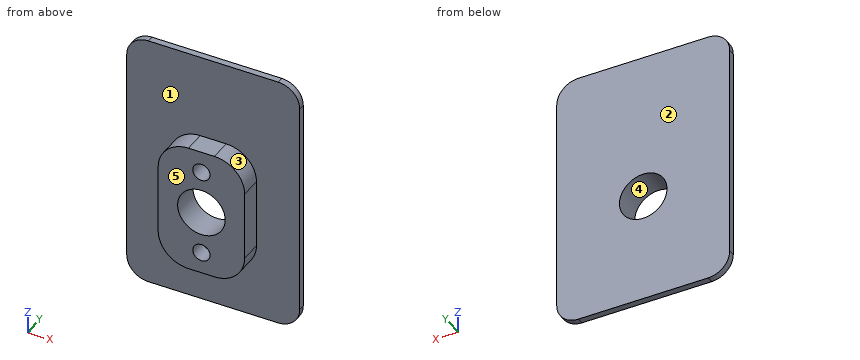
```python
from build123d import *

# Parameters (mm, degrees)
F0_W     = 40
F0_H     = 60
F0_R     = 5.5
F1_DEPTH = 1.5
F2_W     = 20
F2_H     = 30
F2_R     = 5.5
F3_DEPTH = 5
F4_R     = 2
F5_DEPTH = 4
F6_R     = 7
F7_R     = 5


with BuildPart() as f1:
    # F0 (on Front) → F1 (new body)
    with BuildSketch(Plane.XZ):
        with Locations((0, 4.5)):
            Rectangle(F0_W, F0_H)
        Circle(F0_R, mode=Mode.SUBTRACT)
    extrude(amount=F1_DEPTH)

    # F2 (on face) → F3 (join)
    with BuildSketch(Plane.XZ.offset(1.5)):
        Rectangle(F2_W, F2_H)
        Circle(F2_R, mode=Mode.SUBTRACT)
    extrude(amount=F3_DEPTH)

    # F4 (on face) → F5 (cut)
    with BuildSketch(Plane.XZ.offset(6.5)):
        with Locations((0, 10)):
            Circle(F4_R)
        with Locations((0, -10)):
            Circle(F4_R)
    extrude(amount=-F5_DEPTH, mode=Mode.SUBTRACT)

    # F6
    f6_edges = [f1.edges().sort_by_distance(p)[0] for p in [
        (10, -4, 15),
        (-10, -4, 15),
        (10, -4, -15),
        (-10, -4, -15),
    ]]
    fillet(f6_edges, radius=F6_R)

    # F7
    f7_edges = [f1.edges().sort_by_distance(p)[0] for p in [
        (20, -0.75, 34.5),
        (20, -0.75, -25.5),
        (-20, -0.75, -25.5),
        (-20, -0.75, 34.5),
    ]]
    fillet(f7_edges, radius=F7_R)


solid = f1.part
```
Input: part model. Units: mm. Frame: model coordinates. Face numbers are marked on the shaded views. A direction names the side the tool comes from. Round coordinates to 2 decimals unless told otherwise and drop trailing zeros. Loops run counter-clockwise (first coordinate to the right, second up) from the corner with the lowest first, then second, coordinate; pieces in that order, holes last. Notation, with made-up numbers: (39, 72) - (96, 72) arc R29 cw to (96, 99) - close; hole circle Ø6 at (74.25, -32.75). An arc over 180 degrees is marked (long way). One line per item, written item: value. Start each with the question number.
(1) Section B-B, the plane y = -3.25. Return loops of the section in (x, z).
(2) Access query for the marked faces 1 and 2. Directions: +Z, -Z, +X, -X, +Y, -Y. A direction counts if a zero-diameter tool reaches every point of the face in a straight line with its end or side. Return the directions, or none.
(3) Ray query, line 1 (Z direction, x = 0, y = -3.6); line 2 (Y direction, x = -5, z = 19); line 3 (X direction, y = -4.75, z = 1). Return the intervals inside material, ascending. Write a range as [from, to].
(4) Section D-D, the plane x = -8. Return loops of the section in (y, z).
(5) Draft query along Z for the marked faces 3, 4 and 5. Return one class per face: +Z half, -Z half, draft (parallel to the pull), parting line (faces both ways), or undercut.
(6) Contact query for flat-ended pins moving along their axis: P1, Ø9, axis at x = 0, z = 0, coming from the +Y side; P2, Ø1.5, axis at y = -3.5, z = -2.5, coming from the -X side; P3, Ø2, axis at x = 6.5, y = -3, coming from the -Z side. Output: stop coordinate, or through.
(7) Section A-A, the plane z = 0. Return loops of the section in (x, y).
(8) Section C-C, the plane x = 0. Return loops of the section in (y, z), plus the area to 4 significant figures.
Results below:
1. outline: (-10, -8) arc R7 ccw to (-3, -15) - (3, -15) arc R7 ccw to (10, -8) - (10, 8) arc R7 ccw to (3, 15) - (-3, 15) arc R7 ccw to (-10, 8) - close; hole circle Ø11 at (0, 0); hole circle Ø4 at (0, -10); hole circle Ø4 at (0, 10)
2. face 1: -Y
2. face 2: +Z, -Z, +X, -X, +Y
3. line 1: [-15, -12], [-8, -5.5], [5.5, 8], [12, 15]
3. line 2: [-1.5, 0]
3. line 3: [-10, -5.41], [5.41, 10]
4. outline: (-6.5, -12.9) - (-1.5, -12.9) - (-1.5, -25.5) - (0, -25.5) - (0, 34.5) - (-1.5, 34.5) - (-1.5, 12.9) - (-6.5, 12.9) - close
5. face 3: +Z half
5. face 4: undercut
5. face 5: draft
6. P1: through
6. P2: x = -10
6. P3: z = -14.54
7. outline: (-20, -1.5) - (-10, -1.5) - (-10, -6.5) - (-5.5, -6.5) - (-5.5, 0) - (-20, 0) - close; (5.5, -6.5) - (10, -6.5) - (10, -1.5) - (20, -1.5) - (20, 0) - (5.5, 0) - close
8. outline: (-6.5, -15) - (-1.5, -15) - (-1.5, -25.5) - (0, -25.5) - (0, -5.5) - (-6.5, -5.5) - (-6.5, -8) - (-2.5, -8) - (-2.5, -12) - (-6.5, -12) - close; (-6.5, 5.5) - (0, 5.5) - (0, 34.5) - (-1.5, 34.5) - (-1.5, 15) - (-6.5, 15) - (-6.5, 12) - (-2.5, 12) - (-2.5, 8) - (-6.5, 8) - close
8. area: 136.5 mm^2
